Geometry check sheet. Reference: the model listing, model coordinates, mm. A direction names the side the tool comes from. Coordinates: 2 decimals unless noted, no trailing zeros. Order: outer loops, then holes, each group sorted by start corner. A loop starts at its lowest first (then second) coordinate and runs counter-clockwise, first axis right, second up. Notation, with made-up numbers: M 57,49.25 L 96,49.25 A22 cw 96,66.25 Z; hole C 4.25,-6 d4. An arc over 180 degrees is marked long. One line per item, written item: value. Start each with the question number.
1) Draft check along Y on faces 1 (the cylindrical face through (16.046, 2.727, 8.916)), 2 (the flat face through (8, 0, 3)), 3 (the flat face through (10, 0, 0)). Enter one of: pulls with the +Y half, pulls with the -Y half, needs draft (parallel to the pull), parting line crosses it, or undercut.
2) Sectioned sample at A-A, the plane x = -0.25. Enter the section's corners in (y, z).
3) Go/stop test with flat-tipped pins: P1, Ø4, axis at y = 0, z = 11.5, coming from the -X side; P2, Ø1.5, axis at x = 2.5, y = 2.5, coming from the +Z side; P3, Ø3, axis at y = 2, z = 2, coming from the -X side. Record where each tip stops, or that it passes through.
4) Thickness scan on L1, parallel to Z at x = 3.5, y = 1.75; L2, parallel to Z at x = 16.25, y = -4.5; L3, parallel to Z at x = 5.25, y = 3. Record the ranges inside material, lowest first. Write a range as from..to.
5) Access from +Z, -Z, +X, -X, +Y, -Y to the whole of each face (thin tool, end or side, straight path). Record for faces 4 (the cylindrical face through (16.046, -3.021, 17.727)), 5 (the flat face through (11, 0, -1)), 6 (the cylindrical face through (18.32, -0.04, 0.99)).
6) Sectioned sample at C-C, the plane z = 5. Enter the section's corners in (x, y).
7) Sectioned sample at B-B, the plane x = 4.25. Enter the section's corners in (y, z).
8) Sectioned sample at D-D, the plane y = 1.5. Enter the section's corners in (x, z).
```python
from build123d import *

# Parameters (mm, degrees)
F1_DEPTH = 1
F2_DEPTH = 3
F3_DEPTH = 2
F4_R     = 2.75
F5_DEPTH = 12
F7_ANGLE = 90
F8_R     = 2.75
F9_DEPTH = 5
F10_R    = 0.5


# Not quite as in the source:
# - a feature names something its author has since deleted; it is built from what else it names


with BuildPart() as f1:
    # F0 (on Top) → F1 (new body)
    with BuildSketch(Plane.XY):
        with BuildLine():
            ThreePointArc((1.7856760203, -2.9109424849), (-0.4640879363, -3.3833189899), (-2.5035568051, -2.3225908645))
            Line((-2.5035568051, -2.3225908645), (-2.870109778, -2.6626480921))
            ThreePointArc((-2.870109778, -2.6626480921), (-0.7021528954, -3.8515200001), (1.745866363, -3.5041654702))
            ThreePointArc((1.745866363, -3.5041654702), (2.2390334242, -3.2115345748), (2.6841618804, -2.85))
            Line((2.6841618804, -2.85), (1.7856760203, -2.9109424849))
        make_face()
        with BuildLine():
            ThreePointArc((1.7856760202, 2.910942485), (3.415, 0), (1.7856760203, -2.9109424849))
            Line((1.7856760203, -2.9109424849), (2.6841618804, -2.85))
            ThreePointArc((2.6841618804, -2.85), (3.915, 0), (2.6841618804, 2.85))
            Line((2.6841618803, 2.85), (1.7856760202, 2.910942485))
        make_face()
        with BuildLine():
            ThreePointArc((-2.4179432279, 2.4115919113), (-0.4028376898, 3.391157147), (1.7856760202, 2.910942485))
            Line((1.7856760202, 2.910942485), (2.6841618803, 2.85))
            ThreePointArc((2.6841618804, 2.85), (2.2390334242, 3.2115345748), (1.7458663629, 3.5041654702))
            ThreePointArc((1.7458663629, 3.5041654702), (-0.6323981068, 3.8635861107), (-2.7719612701, 2.7646800388))
            Line((-2.7719612701, 2.7646800388), (-2.4179432279, 2.4115919113))
        make_face()
        with BuildLine():
            Line((16.533754708, -1.9106100332), (2.6841618804, -2.85))
            ThreePointArc((2.6841618804, -2.85), (2.2390334242, -3.2115345748), (1.745866363, -3.5041654702))
            Line((1.745866363, -3.5041654702), (2.6841618804, -3.85))
            Line((2.6841618804, -3.85), (16.6009492353, -2.9083500025))
            ThreePointArc((16.6009492353, -2.9083500025), (19.3191618804, 0), (16.6009492353, 2.9083500025))
            Line((16.6009492353, 2.9083500025), (2.6841618803, 3.85))
            Line((2.6841618803, 3.85), (2.6841618803, 2.85))
            Line((2.6841618803, 2.85), (16.533754708, 1.9106100332))
            ThreePointArc((16.533754708, 1.9106100332), (18.3191618804, 0), (16.533754708, -1.9106100332))
        make_face()
        with BuildLine():
            ThreePointArc((2.6841618804, 2.85), (3.915, 0), (2.6841618804, -2.85))
            Line((2.6841618804, -2.85), (16.533754708, -1.9106100332))
            ThreePointArc((16.533754708, -1.9106100332), (18.3191618804, 0), (16.533754708, 1.9106100332))
            Line((16.533754708, 1.9106100332), (2.6841618803, 2.85))
        make_face()
        with BuildLine():
            ThreePointArc((1.7458663629, 3.5041654702), (2.2390334242, 3.2115345748), (2.6841618804, 2.85))
            Line((2.6841618803, 2.85), (2.6841618803, 3.85))
            Line((2.6841618803, 3.85), (1.7458663629, 3.5041654702))
        make_face()
    extrude(amount=-F1_DEPTH)

    # F0 (on Top) → F2 (join)
    with BuildSketch(Plane.XY):
        with BuildLine():
            ThreePointArc((1.7856760203, -2.9109424849), (-0.4640879363, -3.3833189899), (-2.5035568051, -2.3225908645))
            Line((-2.5035568051, -2.3225908645), (-2.870109778, -2.6626480921))
            ThreePointArc((-2.870109778, -2.6626480921), (-0.7021528954, -3.8515200001), (1.745866363, -3.5041654702))
            ThreePointArc((1.745866363, -3.5041654702), (2.2390334242, -3.2115345748), (2.6841618804, -2.85))
            Line((2.6841618804, -2.85), (1.7856760203, -2.9109424849))
        make_face()
        with BuildLine():
            ThreePointArc((1.7856760202, 2.910942485), (3.415, 0), (1.7856760203, -2.9109424849))
            Line((1.7856760203, -2.9109424849), (2.6841618804, -2.85))
            ThreePointArc((2.6841618804, -2.85), (3.915, 0), (2.6841618804, 2.85))
            Line((2.6841618803, 2.85), (1.7856760202, 2.910942485))
        make_face()
        with BuildLine():
            ThreePointArc((-2.4179432279, 2.4115919113), (-0.4028376898, 3.391157147), (1.7856760202, 2.910942485))
            Line((1.7856760202, 2.910942485), (2.6841618803, 2.85))
            ThreePointArc((2.6841618804, 2.85), (2.2390334242, 3.2115345748), (1.7458663629, 3.5041654702))
            ThreePointArc((1.7458663629, 3.5041654702), (-0.6323981068, 3.8635861107), (-2.7719612701, 2.7646800388))
            Line((-2.7719612701, 2.7646800388), (-2.4179432279, 2.4115919113))
        make_face()
        with BuildLine():
            ThreePointArc((1.7458663629, 3.5041654702), (2.2390334242, 3.2115345748), (2.6841618804, 2.85))
            Line((2.6841618803, 2.85), (2.6841618803, 3.85))
            Line((2.6841618803, 3.85), (1.7458663629, 3.5041654702))
        make_face()
        with BuildLine():
            Line((16.533754708, -1.9106100332), (2.6841618804, -2.85))
            ThreePointArc((2.6841618804, -2.85), (2.2390334242, -3.2115345748), (1.745866363, -3.5041654702))
            Line((1.745866363, -3.5041654702), (2.6841618804, -3.85))
            Line((2.6841618804, -3.85), (16.6009492353, -2.9083500025))
            ThreePointArc((16.6009492353, -2.9083500025), (19.3191618804, 0), (16.6009492353, 2.9083500025))
            Line((16.6009492353, 2.9083500025), (2.6841618803, 3.85))
            Line((2.6841618803, 3.85), (2.6841618803, 2.85))
            Line((2.6841618803, 2.85), (16.533754708, 1.9106100332))
            ThreePointArc((16.533754708, 1.9106100332), (18.3191618804, 0), (16.533754708, -1.9106100332))
        make_face()
        with BuildLine():
            ThreePointArc((2.6841618804, 2.85), (3.915, 0), (2.6841618804, -2.85))
            Line((2.6841618804, -2.85), (16.533754708, -1.9106100332))
            ThreePointArc((16.533754708, -1.9106100332), (18.3191618804, 0), (16.533754708, 1.9106100332))
            Line((16.533754708, 1.9106100332), (2.6841618803, 2.85))
        make_face()
    extrude(amount=F2_DEPTH)

    # F0 (on Top) → F3 (cut)
    with BuildSketch(Plane.XY):
        with BuildLine():
            ThreePointArc((2.6841618804, 2.85), (3.915, 0), (2.6841618804, -2.85))
            Line((2.6841618804, -2.85), (16.533754708, -1.9106100332))
            ThreePointArc((16.533754708, -1.9106100332), (18.3191618804, 0), (16.533754708, 1.9106100332))
            Line((16.533754708, 1.9106100332), (2.6841618803, 2.85))
        make_face()
        with BuildLine():
            ThreePointArc((1.7856760202, 2.910942485), (3.415, 0), (1.7856760203, -2.9109424849))
            Line((1.7856760203, -2.9109424849), (2.6841618804, -2.85))
            ThreePointArc((2.6841618804, -2.85), (3.915, 0), (2.6841618804, 2.85))
            Line((2.6841618803, 2.85), (1.7856760202, 2.910942485))
        make_face()
    extrude(amount=F3_DEPTH, mode=Mode.SUBTRACT)

    # F4 (on face) → F5 (join)
    with BuildSketch(Plane.XY.offset(3)):
        with Locations((16.4041618804, 0)):
            Circle(F4_R)
    extrude(amount=F5_DEPTH)

    # F6 (on face) → F7 (revolve)
    with BuildSketch(Plane.XY.offset(15)):
        with BuildLine():
            Line((13.6541618804, 0), (19.1541618804, 0))
            ThreePointArc((19.1541618804, 0), (16.4041618804, 2.75), (13.6541618804, 0))
        make_face()
    revolve(axis=Axis((16.4041618804, 0, 15), (1, 0, 0)), revolution_arc=F7_ANGLE)

    # F8 (on face) → F9 (join)
    with BuildSketch(Plane.XZ):
        with Locations((16.4041618804, 15)):
            Circle(F8_R)
    extrude(amount=F9_DEPTH)

    # F10
    f10_edges = [f1.edges().sort_by_distance(p)[0] for p in [
        (18.503226, -1.776634, 13.223366),
        (14.305098, -1.776634, 13.223366),
    ]]
    fillet(f10_edges, radius=F10_R)


solid = f1.part
```
Final values:
1. face 1: parting line crosses it
1. face 2: needs draft
1. face 3: undercut
2. outline: M -3.91,-1 L -3.41,-1 L -3.41,3 L -3.91,3 Z; M 3.41,-1 L 3.91,-1 L 3.91,3 L 3.41,3 Z
3. P1: stops at x = 13.65
3. P2: stops at z = 3
3. P3: stops at x = -2.77
4. L1: z = -1..0, 2..3
4. L2: z = 12.25..17.75
4. L3: z = -1..3
5. face 4: -Y
5. face 5: -Z, +X, -X, +Y, -Y
5. face 6: -X
6. outline: C 16.4,0 d5.5
7. outline: M -3.74,-1 L 3.74,-1 L 3.74,3 L -3.74,3 Z; hole M -2.74,0 L 2.74,0 L 2.74,2 L -2.74,2 Z
8. outline: M 3.07,-1 L 18.9,-1 L 18.9,3 L 18.71,3 L 18.71,15 A2.3 ccw 14.1,15 L 14.1,3 L 3.07,3 L 3.07,2 L 17.59,2 L 17.59,0 L 3.07,0 Z
